Read the model definition and answer for the solid it produces. Units are mm, in the model's axes. Round coordinates to 2 decimals unless told otherwise and drop trailing zeros. Order: outer loops, then holes, each group sorted by start corner. A loop starts at its lowest first (then second) coordinate and runs counter-clockwise, first axis right, second up. Notation, with made-up numbers: M 59.5,-22 L 85.5,-22 A17 cw 85.5,0 Z; hole C -2.75,45.5 d8. An arc over 180 degrees is marked long. Answer as CSV lines item,"result".
```python
from build123d import *

# Parameters (mm, degrees)
SKETCH1_W           = 75
SKETCH1_H           = 100.95000003
BOSS_EXTRUDE1_DEPTH = 6.35
SKETCH3_R           = 2
CUT_EXTRUDE1_DEPTH  = 6.35
SKETCH4_W           = 75
SKETCH4_H           = 3.175
CUT_EXTRUDE2_DEPTH  = 64.20045986
FILLET1_R           = 3.175
SKETCH5_W           = 27.975
SKETCH5_H           = 19.05
CUT_EXTRUDE3_DEPTH  = 64.20045986
FILLET2_R           = 3.175


with BuildPart() as part:
    # Sketch1 → Boss-Extrude1 (new body)
    with BuildSketch(Plane.XY):
        Rectangle(SKETCH1_W, SKETCH1_H)
    extrude(amount=BOSS_EXTRUDE1_DEPTH)

    # Sketch3 → Cut-Extrude1 (cut)
    with BuildSketch(Plane.XY.offset(6.35)):
        with Locations((-27.975, -37.775000015)):
            Circle(SKETCH3_R)
        with Locations((27.975, -37.775000015)):
            Circle(SKETCH3_R)
    extrude(amount=-CUT_EXTRUDE1_DEPTH, mode=Mode.SUBTRACT)

    # Sketch4 → Cut-Extrude2 (cut, through all)
    with BuildSketch(Plane(origin=(0, 0, 0), x_dir=(-1, 0, 0), z_dir=(0, 0, -1))):
        with Locations((0, 48.887500015)):
            Rectangle(SKETCH4_W, SKETCH4_H)
    extrude(amount=-CUT_EXTRUDE2_DEPTH, mode=Mode.SUBTRACT)

    # Fillet1
    fillet1_edges = [part.edges().sort_by_distance(p)[0] for p in [
        (37.5, 47.300000015, 3.175),
        (-37.5, 47.300000015, 3.175),
    ]]
    fillet(fillet1_edges, radius=FILLET1_R)

    # Sketch5 → Cut-Extrude3 (cut, through all)
    with BuildSketch(Plane(origin=(0, 0, 0), x_dir=(-1, 0, 0), z_dir=(0, 0, -1))):
        with Locations((-17.1625, -19.360000015)):
            Rectangle(SKETCH5_W, SKETCH5_H)
        with Locations((17.1625, -19.360000015)):
            Rectangle(SKETCH5_W, SKETCH5_H)
    extrude(amount=-CUT_EXTRUDE3_DEPTH, mode=Mode.SUBTRACT)

    # Fillet2
    fillet2_edges = [part.edges().sort_by_distance(p)[0] for p in [
        (31.15, -28.885000015, 3.175),
        (31.15, -9.835000015, 3.175),
        (3.175, -9.835000015, 3.175),
        (3.175, -28.885000015, 3.175),
        (-3.175, -28.885000015, 3.175),
        (-3.175, -9.835000015, 3.175),
        (-31.15, -9.835000015, 3.175),
        (-31.15, -28.885000015, 3.175),
    ]]
    fillet(fillet2_edges, radius=FILLET2_R)


solid = part.part
```
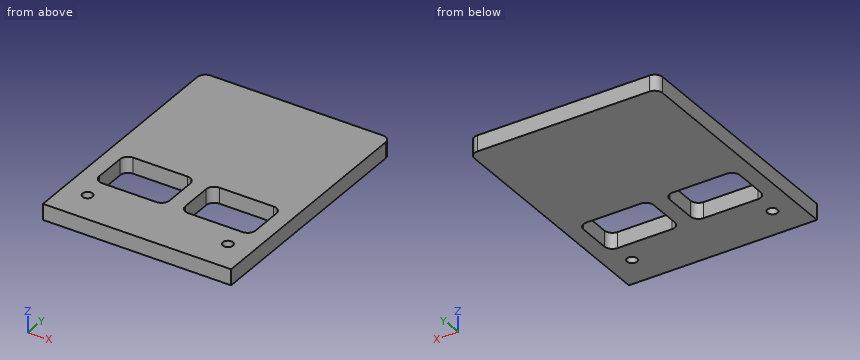
Item 1: Flat-ended cylindrical pins translate along their axes: pin 1 (2.5 mm diameter, centred on x = -27.975, y = -37.775, fed in from +Z); pin 2 (4 mm diameter, centred on x = -21, y = -37.5, fed in from -Z). Find the tip coordinate at first contact, or state that the pin passes through.
Ans:
pin 1,"through"
pin 2,"z = 0"
Item 2: A cutting plane is placed at D-D, the plane x = 5. Determine the outline of the cut face in (y, z) (3 decimals).
Ans:
outline,"M -50.475,0 L -28.584,0 L -28.584,6.35 L -50.475,6.35 Z; M -10.136,0 L 47.3,0 L 47.3,6.35 L -10.136,6.35 Z"
Item 3: A cutting plane is placed at C-C, the plane y = -27. Determine the outline of the cut face in (x, z).
Ans:
outline,"M -37.5,0 L -30.88,0 L -30.88,6.35 L -37.5,6.35 Z; M -3.45,0 L 3.45,0 L 3.45,6.35 L -3.45,6.35 Z; M 30.88,0 L 37.5,0 L 37.5,6.35 L 30.88,6.35 Z"
Item 4: Find the intervals of material crossed by probe 1 along X at (y, z) = (-24, 2.25) (3 decimals); probe 2 along Y at (x, z) = (-8, 1) (3 decimals); probe 3 along X at (y, z) = (-26.5, 4.5), in increasing order. Write a range as [from, to].
Ans:
probe 1,"[-37.5, -31.15], [-3.175, 3.175], [31.15, 37.5]"
probe 2,"[-50.475, -28.885], [-9.835, 47.3]"
probe 3,"[-37.5, -31.05], [-3.27, 3.27], [31.05, 37.5]"
Item 5: A cutting plane is placed at B-B, the plane z = 2. Determine the outline of the cut face in (x, y) (3 decimals), and give its area (3 significant figures).
Ans:
outline,"M -37.5,-50.475 L 37.5,-50.475 L 37.5,44.125 A3.175 ccw 34.325,47.3 L -34.325,47.3 A3.175 ccw -37.5,44.125 Z; hole M -31.15,-25.71 A3.175 ccw -27.975,-28.885 L -6.35,-28.885 A3.175 ccw -3.175,-25.71 L -3.175,-13.01 A3.175 ccw -6.35,-9.835 L -27.975,-9.835 A3.175 ccw -31.15,-13.01 Z; hole C -27.975,-37.775 d4; hole M 3.175,-25.71 A3.175 ccw 6.35,-28.885 L 27.975,-28.885 A3.175 ccw 31.15,-25.71 L 31.15,-13.01 A3.175 ccw 27.975,-9.835 L 6.35,-9.835 A3.175 ccw 3.175,-13.01 Z; hole C 27.975,-37.775 d4"
area,"6,260 mm2"
Item 6: A cutting plane is placed at A-A, the plane x = 24.5. Determine the outline of the cut face in (y, z) (3 decimals).
Ans:
outline,"M -50.475,0 L -28.885,0 L -28.885,6.35 L -50.475,6.35 Z; M -9.835,0 L 47.3,0 L 47.3,6.35 L -9.835,6.35 Z"
